Autodesk Inventor part; units mm, degrees
ref_plane "YZ Plane" through (0, 0, 0) normal (1, 0, 0) x (0, 1, 0)
ref_plane "XZ Plane" through (0, 0, 0) normal (0, 1, 0) x (-1, 0, 0)
ref_plane "XY Plane" through (0, 0, 0) normal (0, 0, 1) x (1, 0, 0)
sketch "Sketch1" plane through (0, 0, 0) normal (0, 1, 0) x (-1, 0, 0)
  line L0 (-5.4993, 0) -> (-2.7496, 4.7625)
  line L1 (-2.7496, 4.7625) -> (2.7496, 4.7625)
  line L2 (2.7496, 4.7625) -> (5.4993, 0)
  line L3 (5.4993, 0) -> (2.7496, -4.7625)
  line L4 (2.7496, -4.7625) -> (-2.7496, -4.7625)
  line L5 (-2.7496, -4.7625) -> (-5.4993, 0)
  circle A0 centre (0, 0) radius 5.125
  point P0 (1.8932, -4.7625)
  point P1 (3.1778, -4.0208)
  point P2 (5.071, -0.7417)
  point P3 (5.071, 0.7417)
  point P4 (3.1778, 4.0208)
  point P5 (1.8932, 4.7625)
  point P6 (-1.8932, 4.7625)
  point P7 (-3.1778, 4.0208)
  point P8 (-5.071, 0.7417)
  point P9 (-5.071, -0.7417)
  point P10 (-3.1778, -4.0208)
  point P11 (-1.8932, -4.7625)
  dimension "d0" = 9.525
  dimension "d1" = 10.25
extrude "Extrusion1" add sketch "Sketch1" along normal blind 60.325 contours L0 A0 L1 L2 L3 L4 L5
sketch "Sketch2" plane through (0, 0, 0) normal (0, -1, 0) x (1, 0, 0)
  circle A0 centre (0, 0) radius 3.175
  arc A1 (3.1778, 4.0208) -> (1.8932, 4.7625) centre (0, 0) ccw
  line L0 (-1.8932, 4.7625) -> (1.8932, 4.7625)
  arc A2 (-1.8932, 4.7625) -> (-3.1778, 4.0208) centre (0, 0) ccw
  line L1 (-5.071, 0.7417) -> (-3.1778, 4.0208)
  arc A3 (-5.071, 0.7417) -> (-5.071, -0.7417) centre (0, 0) ccw
  line L2 (-3.1778, -4.0208) -> (-5.071, -0.7417)
  arc A4 (-3.1778, -4.0208) -> (-1.8932, -4.7625) centre (0, 0) ccw
  line L3 (1.8932, -4.7625) -> (-1.8932, -4.7625)
  arc A5 (1.8932, -4.7625) -> (3.1778, -4.0208) centre (0, 0) ccw
  line L4 (5.071, -0.7417) -> (3.1778, -4.0208)
  arc A6 (5.071, -0.7417) -> (5.071, 0.7417) centre (0, 0) ccw
  line L5 (3.1778, 4.0208) -> (5.071, 0.7417)
  dimension "d4" = 6.35
extrude "Extrusion2" cut sketch "Sketch2" against normal blind 3.175
sketch "Sketch3" plane through (0, 60.325, 0) normal (0, 1, 0) x (1, 0, 0)
  line L0 (5.071, 0.7417) -> (3.1778, 4.0208)
  arc A0 (3.1778, 4.0208) -> (1.8932, 4.7625) centre (0, 0) ccw
  line L1 (1.8932, 4.7625) -> (-1.8932, 4.7625)
  arc A1 (-1.8932, 4.7625) -> (-3.1778, 4.0208) centre (0, 0) ccw
  line L2 (-3.1778, 4.0208) -> (-5.071, 0.7417)
  arc A2 (-5.071, 0.7417) -> (-5.071, -0.7417) centre (0, 0) ccw
  line L3 (-5.071, -0.7417) -> (-3.1778, -4.0208)
  arc A3 (-3.1778, -4.0208) -> (-1.8932, -4.7625) centre (0, 0) ccw
  line L4 (-1.8932, -4.7625) -> (1.8932, -4.7625)
  arc A4 (1.8932, -4.7625) -> (3.1778, -4.0208) centre (0, 0) ccw
  line L5 (3.1778, -4.0208) -> (5.071, -0.7417)
  arc A5 (5.071, -0.7417) -> (5.071, 0.7417) centre (0, 0) ccw
  circle A6 centre (0, 0) radius 3.175
  dimension "d7" = 6.35
extrude "Extrusion3" cut sketch "Sketch3" against normal blind 6.35
properties part number "DriveShaft" material "Steel, Alloy"
Check sheet for the modelled part. Datum: model origin and axes. Units: mm. A direction names the side the tool comes from. Round coordinates to 2 decimals unless told otherwise and drop trailing zeros. Write each loop counter-clockwise with the first axis right and the second up, starting at its lowest first coordinate (ties: lowest second). Pieces come first, ordered by that corner, then holes. Notation, with made-up numbers: (-38.75, 13) -> (5.25, 13) arc R19 cw to (5.25, 26) -> close; hole circle Ø3 at (49, 14). An arc over 180 degrees is marked (long way). Answer as CSV lines item,"result". Start each with the question number.
1) Section check D-D on x = -4. Enter the section's corners in (y, z) (3 decimals).
2) Release check for a two-part mould opening along X. For faces 4 (the flat face through (0, 28, 4.762)), 5 (the flat face through (4.138, 28.219, 2.358)), 6 (the cylindrical face through (-0.69, 57.19, 3.1)) record: pulls with the +X half, pulls with the -X half, needs draft (parallel to the pull), parting line crosses it, or undercut.
3) Material ranges on line 1 (X direction, y = 40.5, z = -0.25); line 2 (Y direction, x = 0, z = -3.5) (3 decimals); line 3 (Z direction, x = -3, y = 6.5), recorded low to high. Write a range as from..to.
4) Go/stop test with a flat-tipped pin: P1, Ø1, axis at y = 27.5, z = 3.5, coming from the -X side. Record where the tip stops, or that it passes through.
5) Section check A-A on x = 0. Enter the section's corners in (y, z) (1 decimal).
6) Tool access check on faces 1 (the cylindrical face through (2.553, 28.219, -4.444)), 2 (the flat face through (-1.2, 53.975, -3.2)), 3 (the flat face through (-1.2, 3.175, 3.2)). Record the directions out of +Z, -Z, +X, -X, +Y, -Y that give a thin tool (end or side, any length) a straight path to the whole face; none if there is none.
7) Section check C-C on x = 4.25. Enter the section's corners in (y, z) (3 decimals), and give its area (3 significant figures).
Found:
1,outline,"(3.175, -2.597) -> (53.975, -2.597) -> (53.975, 2.597) -> (3.175, 2.597) -> close"
2,face 4,"needs draft"
2,face 5,"pulls with the +X half"
2,face 6,"parting line crosses it"
3,line 1,"x = -5.12..5.12"
3,line 2,"y = 3.175..53.975"
3,line 3,"z = -4.16..4.16"
4,P1,"stops at x = -3.77"
5,outline,"(0, -3.2) -> (3.2, -3.2) -> (3.2, -4.8) -> (54, -4.8) -> (54, -3.2) -> (60.3, -3.2) -> (60.3, 3.2) -> (54, 3.2) -> (54, 4.8) -> (3.2, 4.8) -> (3.2, 3.2) -> (0, 3.2) -> close"
6,face 1,"-Z, +X, +Y, -Y"
6,face 2,"+Y"
6,face 3,"-Y"
7,outline,"(3.175, -2.164) -> (53.975, -2.164) -> (53.975, 2.164) -> (3.175, 2.164) -> close"
7,area,"220 mm^2"
